Read the model definition and answer for the solid it produces. Units are mm, in the model's axes. Face numbers are marked on the shaded views. A direction names the side the tool comes from. Round coordinates to 2 decimals unless told otherwise and drop trailing zeros. Write each loop counter-clockwise with the first axis right and the second up, starting at its lowest first coordinate (ties: lowest second). Pieces come first, ordered by that corner, then holes. Notation, with made-up numbers: (-4.5, -32.75) - (34.5, -32.75) arc R18 cw to (34.5, -28.75) - close; hole circle Ø4 at (-20.75, 17). An arc over 180 degrees is marked (long way). Use one line per item in the form item = value. Start each with the question number.
1) For the marked faces 4 and 5, determine the directions among +Z, -Z, +X, -X, +Y, -Y from which every point of the face is accessible in a straight line to the end or side of a thin tool.
2) Consider line 1 along Z through (x, y) = (0, -7) (3 decimals); line 2 along X through (y, z) = (-21, -2); line 3 along Z through (x, y) = (10, -11). Determine where each line is inside the solid, lowest interval first. Write a range as from..to.
3) The part is cut by section C-C, the plane y = -13. Count the separate pieces of the cut face and the enclosed holes in it, plus the area to 3 significant figures.
4) Each of these flat-tipped pins is pushed along its axis until it touches: pin 1 (6.5 mm diameter, centred on x = 10.29, z = 10.03, fed in from -Y); pin 2 (2 mm diameter, centred on y = -15, z = -12.5, fed in from -X); pin 3 (10 mm diameter, centred on y = -1, z = -4, fed in from -X); pin 4 (5 mm diameter, centred on y = -18, z = -24, fed in from -X). Where does it stop, or does it pass through?
5) For a pull along Z with two mould halves and no side action, classify the marked faces 1, 2 and 3 as released by +Z, released by -Z, zero draft, split by the parting line, or undercut.
6) The part is cut by section D-D, the plane x = 32.5. Give the vertices of the cut face in (y, z).
7) The part is cut by section B-B, the plane x = 0. Give the vertices of the cut face in (y, z) (3 decimals), plus the area to 3 significant figures.
8) The part is cut by section A-A, the plane z = 0. Give the vertices of the cut face in (x, y).
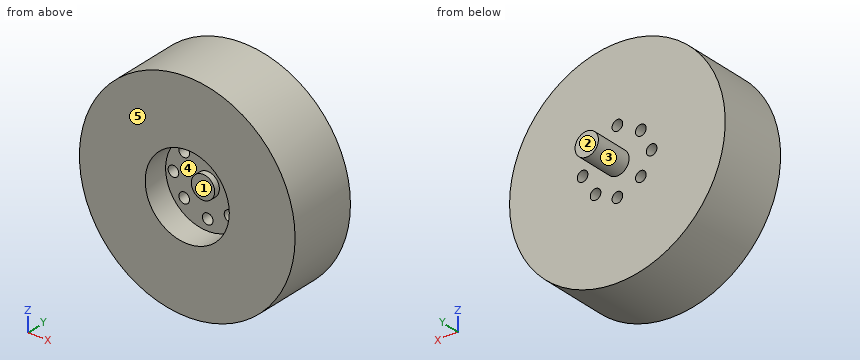
from build123d import *

# Parameters (mm, degrees)
F0_R     = 50.8
F1_DEPTH = 33.02
F2_R     = 19.812
F3_DEPTH = 12.192
F4_R     = 5.5
F5_DEPTH = 2.794
F6_R     = 2.5
F7_DEPTH = 25.4
F8_R     = 5.5
F9_DEPTH = 18.288


with BuildPart() as f1:
    # F0 (on Front) → F1 (new body)
    with BuildSketch(Plane.XZ):
        Circle(F0_R)
    extrude(amount=F1_DEPTH)

    # F2 (on face) → F3 (cut)
    with BuildSketch(Plane.XZ.offset(33.02)):
        Circle(F2_R)
    extrude(amount=-F3_DEPTH, mode=Mode.SUBTRACT)

    # F4 (on face) → F5 (join)
    with BuildSketch(Plane.XZ.offset(20.828)):
        Circle(F4_R)
    extrude(amount=F5_DEPTH)

    # F6 (on face) → F7 (cut)
    with BuildSketch(Plane.XZ.offset(20.828)):
        with Locations((0, 15.8750005066)):
            Circle(F6_R)
        with Locations((-11.048999615, 10.0330002606)):
            Circle(F6_R)
        with Locations((-16.1290001124, 0)):
            Circle(F6_R)
        with Locations((-11.048999615, -9.5250001177)):
            Circle(F6_R)
        with Locations((0, -14.6050006151)):
            Circle(F6_R)
        with Locations((10.286998935, -9.7789997235)):
            Circle(F6_R)
        with Locations((16.3829997182, 0)):
            Circle(F6_R)
        with Locations((10.286998935, 10.0330002606)):
            Circle(F6_R)
    extrude(amount=-F7_DEPTH, mode=Mode.SUBTRACT)

    # F8 (on face) → F9 (join)
    with BuildSketch(Plane(origin=(0, 0, 0), x_dir=(-1, 0, 0), z_dir=(0, 1, 0))):
        Circle(F8_R)
    extrude(amount=F9_DEPTH)


solid = f1.part
Geometry results:
q1.face_4 = -Y
q1.face_5 = +Z, -Z, +X, -X, -Y
q2.line_1 = -50.8..-17.105, -12.105..13.375, 18.375..50.8
q2.line_2 = -50.76..-19.71, -5.12..5.12, 19.71..50.76
q2.line_3 = -49.81..-12.26, -7.3..7.55, 12.52..49.81
q3.separate_pieces = 1
q3.enclosed_holes = 8
q3.area = 7,950 mm2
q4.pin_1 = -20.83
q4.pin_2 = -49.48
q4.pin_3 = -50.8
q4.pin_4 = -46.03
q5.face_1 = undercut
q5.face_2 = zero draft
q5.face_3 = split by the parting line
q6.outline = (-33.02, -39.04) - (0, -39.04) - (0, 39.04) - (-33.02, 39.04) - close
q7.outline = (-33.02, -50.8) - (0, -50.8) - (0, -17.105) - (-20.828, -17.105) - (-20.828, -19.812) - (-33.02, -19.812) - close; (-33.02, 19.812) - (-20.828, 19.812) - (-20.828, 18.375) - (0, 18.375) - (0, 50.8) - (-33.02, 50.8) - close; (-23.622, -5.5) - (-20.828, -5.5) - (-20.828, -12.105) - (0, -12.105) - (0, -5.5) - (18.288, -5.5) - (18.288, 5.5) - (0, 5.5) - (0, 13.375) - (-20.828, 13.375) - (-20.828, 5.5) - (-23.622, 5.5) - close
q7.area = 2,900 mm2
q8.outline = (-50.8, -33.02) - (-19.81, -33.02) - (-19.81, -20.83) - (-18.63, -20.83) - (-18.63, 0) - (-50.8, 0) - close; (-13.63, -20.83) - (-5.5, -20.83) - (-5.5, -23.62) - (5.5, -23.62) - (5.5, -20.83) - (13.88, -20.83) - (13.88, 0) - (5.5, 0) - (5.5, 18.29) - (-5.5, 18.29) - (-5.5, 0) - (-13.63, 0) - close; (18.88, -20.83) - (19.81, -20.83) - (19.81, -33.02) - (50.8, -33.02) - (50.8, 0) - (18.88, 0) - close
